Check sheet for the modelled part. Datum: model origin and axes. Units: mm. Face numbers are marked on the shaded views. Coordinates: 2 decimals unless noted, no trailing zeros. Order: outer loops, then holes, each group sorted by start corner. A loop starts at its lowest first (then second) coordinate and runs counter-clockwise, first axis right, second up.
1. Cross-section at A-A (x = 0). Enter the section's corners in (y, z).
2. Cross-section at B-B (y = 0). Enter the section's corners in (x, z).
3. Cross-section at D-D (z = 12.25). Enter the section's corners in (x, y), then the cut area to 3 significant figures.
4. Cross-section at C-C (z = 22.75). Enter the section's corners in (x, y).
5. Draft check along Z on the marked faces 1, 2, 3 and 4. Enter one of: released by +Z, released by -Z, zero draft, split by the parting line, or undercut.
6. Gauge pin test, flat ends, axial feed: pin 1 Ø4 at (x, y) = (0, -0.5) entering from +Z; pin 2 Ø1.2 at (x, y) = (0, 0.5) entering from +Z; pin 3 Ø3 at (x, z) = (0, 5) entering from +Y; pin 4 Ø2 at (x, z) = (-2, 15) entering from -Y. Record the tip position at first contact, or that the pin passes through.
7. Thickness scan on line 1 (Z direction, x = 0, y = 1); line 2 (Z direction, x = 0, y = 3.25); line 3 (Y direction, x = 0, z = 26.5). Record the ranges inside material, lowest first.
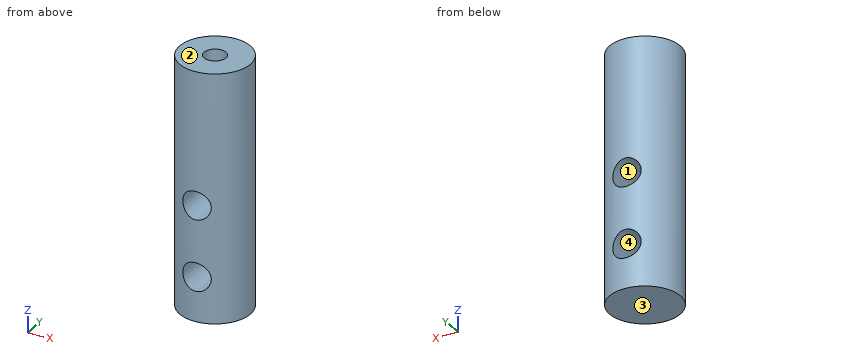
```python
from build123d import *

# Parameters (mm, degrees)
SKETCH_311_R          = 4
EXTRUDE_356_DEPTH     = 28
SKETCH_440_R          = 1.6
CUT_EXTRUDE_537_DEPTH = 30.393876913
SKETCH_1_R            = 1.25
CUT_EXTRUDE_1_DEPTH   = 8


with BuildPart() as part:
    # Sketch 311 → Extrude 356 (new body)
    with BuildSketch(Plane.XY):
        Circle(SKETCH_311_R)
    extrude(amount=EXTRUDE_356_DEPTH)

    # Sketch 440 → Cut-Extrude 537 (cut, through all)
    with BuildSketch(Plane(origin=(0, 4, 0), x_dir=(1, 0, 0), z_dir=(0, 1, 0))):
        with Locations(Location((0, -5, 0), (0, 0, 270))):
            Circle(SKETCH_440_R)
        with Locations(Location((0, -13, 0), (0, 0, 270))):
            Circle(SKETCH_440_R)
    extrude(amount=-CUT_EXTRUDE_537_DEPTH, mode=Mode.SUBTRACT)

    # Sketch 1 → Cut-Extrude 1 (cut)
    with BuildSketch(Plane.XY.offset(28)):
        Circle(SKETCH_1_R)
    extrude(amount=-CUT_EXTRUDE_1_DEPTH, mode=Mode.SUBTRACT)


solid = part.part
```
Data:
1. outline: (-4, 0) - (4, 0) - (4, 3.4) - (-4, 3.4) - close; (-4, 6.6) - (4, 6.6) - (4, 11.4) - (-4, 11.4) - close; (-4, 14.6) - (4, 14.6) - (4, 28) - (1.25, 28) - (1.25, 20) - (-1.25, 20) - (-1.25, 28) - (-4, 28) - close
2. outline: (-4, 0) - (4, 0) - (4, 28) - (1.25, 28) - (1.25, 20) - (-1.25, 20) - (-1.25, 28) - (-4, 28) - close; hole circle Ø3.2 at (0, 5); hole circle Ø3.2 at (0, 13)
3. outline: (-1.41, -3.74) - (-1.41, 3.74) arc R4 ccw to start; (1.41, -3.74) arc R4 ccw to (1.41, 3.74) - close
3. area: 28.1 mm2
4. outline: circle Ø8 at (0, 0); hole circle Ø2.5 at (0, 0)
5. face 1: undercut
5. face 2: released by +Z
5. face 3: released by -Z
5. face 4: undercut
6. pin 1: stops at z = 28
6. pin 2: stops at z = 20
6. pin 3: passes through
6. pin 4: stops at y = -3.87
7. line 1: z = 0 to 3.4, 6.6 to 11.4, 14.6 to 20
7. line 2: z = 0 to 3.4, 6.6 to 11.4, 14.6 to 28
7. line 3: y = -4 to -1.25, 1.25 to 4
